The drawing under review shows one solid part. Ordinate dimensions are in mm from its lowest x, y, z. Coordinates: 2 decimals unless noted, no trailing zeros. Order: outer loops, then holes, each group sorted by start corner. A loop starts at its lowest first (then second) coordinate and runs counter-clockwise, first axis right, second up. Notation, with made-up numbers: (-13.5, 47) -> (32.5, 47) arc R26 ccw to (32.5, 67) -> close; hole circle Ø10 at (-22.5, 54.5). An arc over 180 degrees is marked (long way). Write item = value, one per line.
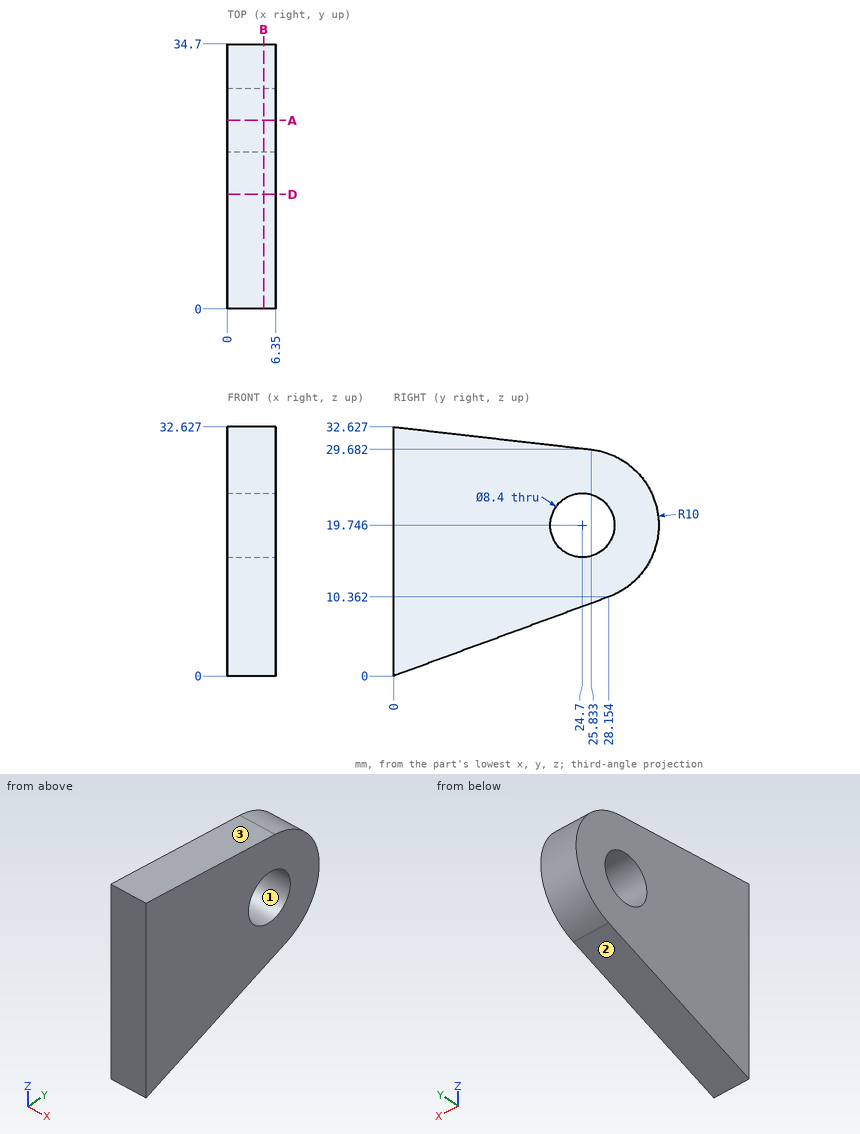
(1) We need section B-B (x = 4.75). Write out the cut boundary in (y, z).
Report:
outline = (0, 0) -> (28.15, 10.36) arc R10 ccw to (25.83, 29.68) -> (0, 32.63) -> close; hole circle Ø8.4 at (24.7, 19.75)
(2) Insertion check: pin 1 (3 mm diameter, centred on x = 1.5, z = 13.5, fed in from +Y); pin 2 (1.5 mm diameter, centred on x = 3, z = 16, fed in from +Y). Each pin has a flat end and moves straight along its axis. Give the tip position at first contact, or say it passes through.
Report:
pin_1 = 33.5
pin_2 = 34.24
(3) We need section A-A (y = 24.7). Write out the cut boundary in (x, z).
Report:
outline = (0, 9.09) -> (6.35, 9.09) -> (6.35, 15.55) -> (0, 15.55) -> close; (0, 23.95) -> (6.35, 23.95) -> (6.35, 29.81) -> (0, 29.81) -> close
(4) For L1, parallel to Z at x = 2, y = 24.7 (1 decimal); L2, parallel to Y at x = 0.5, z = 23 (1 decimal); L3, parallel to Y at x = 2.25, z = 19, list the stretches that pass through material, from the lowest coordinate up.
Report:
L1 = 9.1 to 15.5, 23.9 to 29.8
L2 = 0 to 22, 27.4 to 34.2
L3 = 0 to 20.57, 28.83 to 34.67
(5) We need section D-D (y = 15). Write out the cut boundary in (x, z).
Report:
outline = (0, 5.52) -> (6.35, 5.52) -> (6.35, 30.92) -> (0, 30.92) -> close
(6) The part is to be moulded in two halves that separate along Z. For the marked faces 1, 2 and 3, say which applies: released by +Z, released by -Z, zero draft, split by the parting line, or undercut.
Report:
face_1 = undercut
face_2 = released by -Z
face_3 = released by +Z
